Model file for the job. Use its own axes, mm. Face numbers are marked on the shaded views. A direction names the side the tool comes from. Give positions to 0.01 mm unless a question says otherwise; leave off trailing zeros. Order: outer loops, then holes, each group sorted by start corner. A loop starts at its lowest first (then second) coordinate and runs counter-clockwise, first axis right, second up. Notation, with made-up numbers: (17.5, -24) -> (23.5, -24) arc R9 ccw to (23.5, -13) -> close; hole circle Ø9 at (27.5, 42). An arc over 180 degrees is marked (long way). Answer in a Markdown table with one row per item. Add a question column.
from build123d import *

# Parameters (mm, degrees)
SKETCH1_W           = 10
SKETCH1_H           = 8.2
BOSS_EXTRUDE1_DEPTH = 4.2
CUT_EXTRUDE1_DEPTH  = 10
CUT_EXTRUDE2_DEPTH  = 10
CUT_EXTRUDE4_DEPTH  = 4.7
CUT_EXTRUDE5_REACH  = 6.2
SKETCH6_W           = 8.1
SKETCH6_H           = 2.5


with BuildPart() as part:
    # Sketch1 → Boss-Extrude1 (new body)
    with BuildSketch(Plane(origin=(0, 0, 0), x_dir=(1, 0, 0), z_dir=(0, 1, 0))):
        with Locations((5, -4.1)):
            Rectangle(SKETCH1_W, SKETCH1_H)
    extrude(amount=BOSS_EXTRUDE1_DEPTH)

    # Sketch2 → Cut-Extrude1 (cut)
    with BuildSketch(Plane.ZY):
        Polygon((8.2, 4.2), (8.2, 1.6), (5.7, 1.94), (5.7, 4.2), align=None)
    extrude(amount=-CUT_EXTRUDE1_DEPTH, mode=Mode.SUBTRACT)

    # Sketch3 → Cut-Extrude2 (cut)
    with BuildSketch(Plane.ZY):
        Polygon((0, 2.414814815), (4.7, 2.414814815), (4.7, 2.714814815), (2, 2.914814815), (1.985185185, 2.714814815), (1.485185185, 2.714814815), (1, 3.2), (1, 4.2), (0, 4.2), align=None)
    extrude(amount=-CUT_EXTRUDE2_DEPTH, mode=Mode.SUBTRACT)

    # Sketch4 → Cut-Extrude4 (cut)
    with BuildSketch(Plane(origin=(0, 0, 0), x_dir=(-1, 0, 0), z_dir=(0, 0, -1))):
        Polygon((-9.65, 0.93347747), (-9.65, 1.674146142), (-9.05, 1.674146142), (-9.05, 4.2), (-0.95, 4.2), (-0.95, 1.674146142), (-0.35, 1.674146142), (-0.35, 0.93347747), align=None)
    extrude(amount=-CUT_EXTRUDE4_DEPTH, mode=Mode.SUBTRACT)

    # Cut-Extrude5: up to this face of the body (flat: up to its plane)
    cut_extrude5_end = Plane(part.part.faces().sort_by_distance((5, 1.77, 6.95))[0])
    # Sketch6 → Cut-Extrude5 (cut, up to the picked face)
    with BuildSketch(Plane.XZ, mode=Mode.PRIVATE) as cut_extrude5_sk1:
        with Locations((5, 6.95)):
            Rectangle(SKETCH6_W, SKETCH6_H)
    cut_extrude5_tool1 = split(extrude(cut_extrude5_sk1.sketch, amount=-CUT_EXTRUDE5_REACH, mode=Mode.PRIVATE), bisect_by=cut_extrude5_end, keep=Keep.BOTH, mode=Mode.PRIVATE)
    add(cut_extrude5_tool1.solids().sort_by_distance((5, 0, 6.95))[0], mode=Mode.SUBTRACT)


solid = part.part
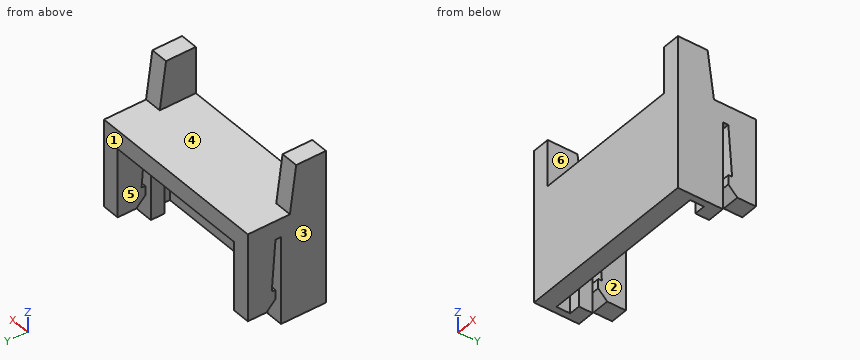
Item 1: Saw through at B-B on y = 3.7. List the corners of the cut face in (x, z).
Item 2: Saw through at D-D on x = 2.5. List the corners of the cut face in (y, z).
Item 3: Pin check, flat tips, straight feed: pin 1 Ø0.5 at (x, z) = (9, 2.5) entering from -Y; pin 2 Ø0.8 at (x, y) = (9.5, 4) entering from -Z; pin 3 Ø3 at (x, z) = (3.5, 3) entering from +Y; pin 4 Ø1.3 at (x, y) = (5.5, 2.5) entering from +Z. Stop position of each tip, or through.
Item 4: Which spindle directions (+Z, -Z, +X, -X, +Y, -Y) get a long thin tool onto all of the face, cutting with end or side? Do the marked faces 4, 5 and 6. Say none if no direction does.
Item 5: Wall check: line 1 (X direction, y = 3.15, z = 3.25); line 2 (Z direction, x = 2, y = 3.9); line 3 (Z direction, x = 5.75, y = 0.4). Give the ranges that are in metal, low to high.
Item 6: Saw through at A-A on z = 3.75. List the corners of the cut face in (x, y), plus the area to 3 significant figures.
Item 7: Saw through at C-C on z = 7.5. List the corners of the cut face in (x, y).
Item 8: Two-plate mould, pull along X, no slides. Class the marked faces 1, 2 and 3: pulls with the +X half, pulls with the -X half, needs draft (parallel to the pull), parting line crosses it, or undercut.
Evaluation:
| question | item | result |
|---|---|---|
| 1 | outline | (0, 1) -> (0.95, 1) -> (0.95, 4.7) -> (9.05, 4.7) -> (9.05, 1) -> (10, 1) -> (10, 5.7) -> (0, 5.7) -> close |
| 2 | outline | (0, 0) -> (0.93, 0) -> (0.93, 4.7) -> (4.2, 4.7) -> (4.2, 5.7) -> (0, 5.7) -> close |
| 3 | pin 1 | stops at y = 0 |
| 3 | pin 2 | stops at z = 1 |
| 3 | pin 3 | stops at y = 0.93 |
| 3 | pin 4 | stops at z = 5.7 |
| 4 | face 4 | +Z, +Y |
| 4 | face 5 | -Z, +Y |
| 4 | face 6 | +Z, +Y, -Y |
| 5 | line 1 | x = 0 to 0.95, 9.05 to 10 |
| 5 | line 2 | z = 4.7 to 5.7 |
| 5 | line 3 | z = 0 to 5.7 |
| 6 | outline | (0, 0) -> (10, 0) -> (10, 2.41) -> (9.05, 2.41) -> (9.05, 1.67) -> (9.65, 1.67) -> (9.65, 0.93) -> (0.35, 0.93) -> (0.35, 1.67) -> (0.95, 1.67) -> (0.95, 2.41) -> (0, 2.41) -> close; (0, 2.79) -> (0.95, 2.79) -> (0.95, 4.2) -> (0, 4.2) -> close; (9.05, 2.79) -> (10, 2.79) -> (10, 4.2) -> (9.05, 4.2) -> close |
| 6 | area | 13.9 mm2 |
| 7 | outline | (0, 0) -> (0.95, 0) -> (0.95, 1.7) -> (0, 1.7) -> close; (9.05, 0) -> (10, 0) -> (10, 1.7) -> (9.05, 1.7) -> close |
| 8 | face 1 | needs draft |
| 8 | face 2 | undercut |
| 8 | face 3 | pulls with the -X half |
